Source: CAD feature listing. Evaluate the final solid. Frame: model axes, mm. A direction names the side the tool comes from. Coordinates: 2 decimals unless noted, no trailing zeros. Loops run counter-clockwise (first coordinate to the right, second up) from the corner with the lowest first, then second, coordinate; pieces in that order, holes last.
Item 1: Section query C-C, the plane z = 26.5. Return the cut outline in (x, y).
Item 2: Section query B-B, the plane y = 0. Return the cut outline in (x, z), then the cut area to 3 significant figures.
Item 3: Pin query (flat end, axial travel): pin 1 Ø3 at (x, z) = (20, -9.5) entering from -Y; pin 2 Ø2.5 at (x, z) = (4.5, -31) entering from +Y; pin 3 Ø10.5 at (x, z) = (30, -27.5) entering from -Y. Return the tip coordinate at first contact, or that it passes through.
Item 4: Line query: probe 1 along Y at (x, z) = (-8.5, 3.5); probe 2 along Z at (x, y) = (19, -37); probe 3 along Z at (x, y) = (41.5, 3.5). Output: solid intervals per line, ascending.
Item 5: Pull-direction query (X, two-part tool) for faces 1 (the cylindrical face through (31.204, 16.167, 45.87)), 2 (the flat face through (14, 10, -32.2)); classes: +X half, -X half, draft (parallel to the pull), parting line (faces both ways), or undercut.
Item 6: Reachability of faces 3 (the cylindrical face through (-13.887, -10.648, 45.87)), 4 (the flat face through (-36, -40, -19.2)), 5 (the cylindrical face through (5.1, -32.15, 37.79)), 6 (the cylindrical face through (15.6, -40.1, 9.2)) from +Z, -Z, +X, -X, +Y, -Y: full face, straight path, thin tool, end or side. Return the list, or none.
Item 7: Section query A-A, the plane y = -22. Return the cut outline in (x, z).
Item 8: Section query D-D, the plane x = 35. State how many separate pieces and enclosed holes the cut face has, then the cut area to 3 significant figures.
```python
from build123d import *

# Parameters (mm, degrees)
BOSS_EXTRUDE1_DEPTH      = 54.4
BOSS_EXTRUDE1_DEPTH_BACK = 45.6
CUT_EXTRUDE1_REACH       = 92
SKETCH3_R                = 3.8
SKETCH3_R_2              = 5
SKETCH3_R_3              = 17.5
SKETCH3_R_4              = 1.7
CUT_EXTRUDE2_REACH       = 92
SKETCH4_R                = 5.1
SKETCH4_R_2              = 5.099999999
SKETCH4_R_3              = 3.4
SKETCH6_W                = 20
SKETCH6_H                = 20
CUT_EXTRUDE4_DEPTH       = 91
SKETCH7_W                = 20
SKETCH7_H                = 20
CUT_EXTRUDE5_DEPTH       = 91
SKETCH5_W                = 3
SKETCH5_H                = 20
SKETCH5_W_2              = 20
SKETCH5_H_2              = 3
CUT_EXTRUDE3_DEPTH       = 101
BOSS_EXTRUDE2_DEPTH      = 80


with BuildPart() as part:
    # Sketch2 → Boss-Extrude1 (new body, two sides)
    with BuildSketch(Plane(origin=(0, 0, 0), x_dir=(0, 0, -1), z_dir=(1, 0, 0))) as boss_extrude1_sk:
        with BuildLine():
            Line((-30.8, -44.997596663), (19.2, -44.997596663))
            ThreePointArc((19.2, -44.997596663), (33.342135624, -39.139732287), (39.2, -24.997596663))
            Line((39.2, -24.997596663), (39.2, 25.002403337))
            ThreePointArc((39.2, 25.002403337), (33.342135624, 39.144538961), (19.2, 45.002403337))
            Line((19.2, 45.002403337), (-30.8, 45.002403337))
            ThreePointArc((-30.8, 45.002403337), (-44.942135624, 39.144538961), (-50.8, 25.002403337))
            Line((-50.8, 25.002403337), (-50.8, -24.997596663))
            ThreePointArc((-50.8, -24.997596663), (-44.942135624, -39.139732287), (-30.8, -44.997596663))
        make_face()
        with BuildLine():
            Line((-30.8, 35.002403337), (19.2, 35.002403337))
            ThreePointArc((19.2, 35.002403337), (26.271067812, 32.073471149), (29.2, 25.002403337))
            Line((29.2, 25.002403337), (29.2, -24.997596663))
            ThreePointArc((29.2, -24.997596663), (26.271067812, -32.068664475), (19.2, -34.997596663))
            Line((19.2, -34.997596663), (-30.8, -34.997596663))
            ThreePointArc((-30.8, -34.997596663), (-37.871067812, -32.068664475), (-40.8, -24.997596663))
            Line((-40.8, -24.997596663), (-40.8, 25.002403337))
            ThreePointArc((-40.8, 25.002403337), (-37.871067812, 32.073471149), (-30.8, 35.002403337))
        make_face(mode=Mode.SUBTRACT)
    extrude(amount=BOSS_EXTRUDE1_DEPTH)
    extrude(boss_extrude1_sk.sketch, amount=-BOSS_EXTRUDE1_DEPTH_BACK)

    # Sketch3 → Cut-Extrude1 (cut, up to next)
    with BuildSketch(Plane.XY.offset(50.8), mode=Mode.PRIVATE) as cut_extrude1_sk1:
        with Locations((35, -16)):
            Circle(SKETCH3_R)
    cut_extrude1_tool1 = extrude(cut_extrude1_sk1.sketch, amount=-CUT_EXTRUDE1_REACH, mode=Mode.PRIVATE) & part.part
    add(cut_extrude1_tool1.solids().sort_by_distance((35, -16, 50.8))[0], mode=Mode.SUBTRACT)
    # Sketch3 → Cut-Extrude1 (cut, up to next)
    with BuildSketch(Plane.XY.offset(50.8), mode=Mode.PRIVATE) as cut_extrude1_sk2:
        with Locations((35, 0)):
            Circle(SKETCH3_R_2)
    cut_extrude1_tool2 = extrude(cut_extrude1_sk2.sketch, amount=-CUT_EXTRUDE1_REACH, mode=Mode.PRIVATE) & part.part
    add(cut_extrude1_tool2.solids().sort_by_distance((35, 0, 50.8))[0], mode=Mode.SUBTRACT)
    # Sketch3 → Cut-Extrude1 (cut, up to next)
    with BuildSketch(Plane.XY.offset(50.8), mode=Mode.PRIVATE) as cut_extrude1_sk3:
        with Locations((35, 16)):
            Circle(SKETCH3_R)
    cut_extrude1_tool3 = extrude(cut_extrude1_sk3.sketch, amount=-CUT_EXTRUDE1_REACH, mode=Mode.PRIVATE) & part.part
    add(cut_extrude1_tool3.solids().sort_by_distance((35, 16, 50.8))[0], mode=Mode.SUBTRACT)
    # Sketch3 → Cut-Extrude1 (cut, up to next)
    with BuildSketch(Plane.XY.offset(50.8), mode=Mode.PRIVATE) as cut_extrude1_sk4:
        Circle(SKETCH3_R_3)
    cut_extrude1_tool4 = extrude(cut_extrude1_sk4.sketch, amount=-CUT_EXTRUDE1_REACH, mode=Mode.PRIVATE) & part.part
    add(cut_extrude1_tool4.solids().sort_by_distance((0, 0, 50.8))[0], mode=Mode.SUBTRACT)
    # Sketch3 → Cut-Extrude1 (cut, up to next)
    with BuildSketch(Plane.XY.offset(50.8), mode=Mode.PRIVATE) as cut_extrude1_sk5:
        with Locations((15.5, 15.5)):
            Circle(SKETCH3_R_4)
    cut_extrude1_tool5 = extrude(cut_extrude1_sk5.sketch, amount=-CUT_EXTRUDE1_REACH, mode=Mode.PRIVATE) & part.part
    add(cut_extrude1_tool5.solids().sort_by_distance((15.5, 15.5, 50.8))[0], mode=Mode.SUBTRACT)
    # Sketch3 → Cut-Extrude1 (cut, up to next)
    with BuildSketch(Plane.XY.offset(50.8), mode=Mode.PRIVATE) as cut_extrude1_sk6:
        with Locations((15.5, -15.5)):
            Circle(SKETCH3_R_4)
    cut_extrude1_tool6 = extrude(cut_extrude1_sk6.sketch, amount=-CUT_EXTRUDE1_REACH, mode=Mode.PRIVATE) & part.part
    add(cut_extrude1_tool6.solids().sort_by_distance((15.5, -15.5, 50.8))[0], mode=Mode.SUBTRACT)
    # Sketch3 → Cut-Extrude1 (cut, up to next)
    with BuildSketch(Plane.XY.offset(50.8), mode=Mode.PRIVATE) as cut_extrude1_sk7:
        with Locations((-15.5, 15.5)):
            Circle(SKETCH3_R_4)
    cut_extrude1_tool7 = extrude(cut_extrude1_sk7.sketch, amount=-CUT_EXTRUDE1_REACH, mode=Mode.PRIVATE) & part.part
    add(cut_extrude1_tool7.solids().sort_by_distance((-15.5, 15.5, 50.8))[0], mode=Mode.SUBTRACT)
    # Sketch3 → Cut-Extrude1 (cut, up to next)
    with BuildSketch(Plane.XY.offset(50.8), mode=Mode.PRIVATE) as cut_extrude1_sk8:
        with Locations((-15.5, -15.5)):
            Circle(SKETCH3_R_4)
    cut_extrude1_tool8 = extrude(cut_extrude1_sk8.sketch, amount=-CUT_EXTRUDE1_REACH, mode=Mode.PRIVATE) & part.part
    add(cut_extrude1_tool8.solids().sort_by_distance((-15.5, -15.5, 50.8))[0], mode=Mode.SUBTRACT)

    # Sketch4 → Cut-Extrude2 (cut, up to next)
    with BuildSketch(Plane.XZ.offset(44.997596663), mode=Mode.PRIVATE) as cut_extrude2_sk1:
        with Locations((-15.6, 5.8)):
            Circle(SKETCH4_R)
    cut_extrude2_tool1 = extrude(cut_extrude2_sk1.sketch, amount=-CUT_EXTRUDE2_REACH, mode=Mode.PRIVATE) & part.part
    add(cut_extrude2_tool1.solids().sort_by_distance((-15.6, -44.997597, 5.8))[0], mode=Mode.SUBTRACT)
    # Sketch4 → Cut-Extrude2 (cut, up to next)
    with BuildSketch(Plane.XZ.offset(44.997596663), mode=Mode.PRIVATE) as cut_extrude2_sk2:
        with Locations((19.4, 5.8)):
            Circle(SKETCH4_R_2)
    cut_extrude2_tool2 = extrude(cut_extrude2_sk2.sketch, amount=-CUT_EXTRUDE2_REACH, mode=Mode.PRIVATE) & part.part
    add(cut_extrude2_tool2.solids().sort_by_distance((19.4, -44.997597, 5.8))[0], mode=Mode.SUBTRACT)
    # Sketch4 → Cut-Extrude2 (cut, up to next)
    with BuildSketch(Plane.XZ.offset(44.997596663), mode=Mode.PRIVATE) as cut_extrude2_sk3:
        with Locations((-15.6, 21.8)):
            Circle(SKETCH4_R_3)
    cut_extrude2_tool3 = extrude(cut_extrude2_sk3.sketch, amount=-CUT_EXTRUDE2_REACH, mode=Mode.PRIVATE) & part.part
    add(cut_extrude2_tool3.solids().sort_by_distance((-15.6, -44.997597, 21.8))[0], mode=Mode.SUBTRACT)
    # Sketch4 → Cut-Extrude2 (cut, up to next)
    with BuildSketch(Plane.XZ.offset(44.997596663), mode=Mode.PRIVATE) as cut_extrude2_sk4:
        with Locations((-15.6, -10.2)):
            Circle(SKETCH4_R_3)
    cut_extrude2_tool4 = extrude(cut_extrude2_sk4.sketch, amount=-CUT_EXTRUDE2_REACH, mode=Mode.PRIVATE) & part.part
    add(cut_extrude2_tool4.solids().sort_by_distance((-15.6, -44.997597, -10.2))[0], mode=Mode.SUBTRACT)
    # Sketch4 → Cut-Extrude2 (cut, up to next)
    with BuildSketch(Plane.XZ.offset(44.997596663), mode=Mode.PRIVATE) as cut_extrude2_sk5:
        with Locations((19.4, 21.8)):
            Circle(SKETCH4_R_3)
    cut_extrude2_tool5 = extrude(cut_extrude2_sk5.sketch, amount=-CUT_EXTRUDE2_REACH, mode=Mode.PRIVATE) & part.part
    add(cut_extrude2_tool5.solids().sort_by_distance((19.4, -44.997597, 21.8))[0], mode=Mode.SUBTRACT)
    # Sketch4 → Cut-Extrude2 (cut, up to next)
    with BuildSketch(Plane.XZ.offset(44.997596663), mode=Mode.PRIVATE) as cut_extrude2_sk6:
        with Locations((19.4, -10.2)):
            Circle(SKETCH4_R_3)
    cut_extrude2_tool6 = extrude(cut_extrude2_sk6.sketch, amount=-CUT_EXTRUDE2_REACH, mode=Mode.PRIVATE) & part.part
    add(cut_extrude2_tool6.solids().sort_by_distance((19.4, -44.997597, -10.2))[0], mode=Mode.SUBTRACT)

    # Sketch6 → Cut-Extrude4 (cut, through all)
    with BuildSketch(Plane(origin=(0, 0, -39.2), x_dir=(-1, 0, 0), z_dir=(0, 0, -1))):
        with Locations((35.6, 35.002403337)):
            Rectangle(SKETCH6_W, SKETCH6_H)
    extrude(amount=-CUT_EXTRUDE4_DEPTH, mode=Mode.SUBTRACT)

    # Sketch7 → Cut-Extrude5 (cut, through all)
    with BuildSketch(Plane.XZ.offset(44.997596663)):
        with Locations((-35.6, -29.2)):
            Rectangle(SKETCH7_W, SKETCH7_H)
    extrude(amount=-CUT_EXTRUDE5_DEPTH, mode=Mode.SUBTRACT)

    # Sketch5 → Cut-Extrude3 (cut, through all)
    with BuildSketch(Plane.ZY.offset(45.6)):
        Polygon((-29.2, 25.002403337), (-19.2, 25.002403337), (-19.2, 35.002403337), (-19.2, 38.002403337), (-19.2, 45.002403337), (-39.2, 45.002403337), (-39.2, 25.002403337), (-32.2, 25.002403337), align=None)
        with Locations((-30.7, 15.002403337)):
            Rectangle(SKETCH5_W, SKETCH5_H)
        with Locations((-9.2, 36.502403337)):
            Rectangle(SKETCH5_W_2, SKETCH5_H_2)
    extrude(amount=-CUT_EXTRUDE3_DEPTH, mode=Mode.SUBTRACT)

    # Sketch8 → Boss-Extrude2 (add)
    with BuildSketch(Plane.ZY.offset(25.6)):
        with BuildLine():
            Line((-19.2, 38.002403337), (-19.2, 25.002403337))
            Line((-19.2, 25.002403337), (-32.2, 25.002403337))
            Line((-32.2, 25.002403337), (-32.2, 15.002403337))
            Line((-32.2, 15.002403337), (-19.2, 15.002403337))
            ThreePointArc((-19.2, 15.002403337), (-12.128932188, 17.931335525), (-9.2, 25.002403337))
            Line((-9.2, 25.002403337), (-9.2, 38.002403337))
            Line((-9.2, 38.002403337), (-19.2, 38.002403337))
        make_face()
    extrude(amount=-BOSS_EXTRUDE2_DEPTH)


solid = part.part
```
Verdict:
1. outline: (-45.6, -45) - (54.4, -45) - (54.4, -35) - (-45.6, -35) - close; (-25.6, 35) - (54.4, 35) - (54.4, 45) - (-25.6, 45) - close
2. outline: (-45.6, 40.8) - (-17.5, 40.8) - (-17.5, 50.8) - (-45.6, 50.8) - close; (-25.6, -39.2) - (54.4, -39.2) - (54.4, -29.2) - (-25.6, -29.2) - close; (17.5, 40.8) - (30, 40.8) - (30, 50.8) - (17.5, 50.8) - close; (40, 40.8) - (54.4, 40.8) - (54.4, 50.8) - (40, 50.8) - close
2. area: 1,350 mm2
3. pin 1: stops at y = 19.28
3. pin 2: stops at y = 25
3. pin 3: stops at y = -44.76
4. probe 1: y = -45 to -35, 35 to 45
4. probe 2: z = -35.2 to -13.58, -6.82 to 0.72, 10.88 to 18.42, 25.18 to 46.8
4. probe 3: z = -39.2 to -29.2, 40.8 to 50.8
5. face 1: undercut
5. face 2: draft
6. face 3: +Z
6. face 4: -Z, -X, +Y, -Y
6. face 5: +X, -X
6. face 6: -Y
7. outline: (-45.6, 40.8) - (54.4, 40.8) - (54.4, 50.8) - (-45.6, 50.8) - close; (-25.6, -39.2) - (54.4, -39.2) - (54.4, -29.2) - (-25.6, -29.2) - close
8. separate pieces: 3
8. enclosed holes: 0
8. area: 2,670 mm2
